Design review of the part built by this model. Coordinates are the model's own, in mm. A direction names the side the tool comes from. Give positions to 0.01 mm unless a question says otherwise; leave off trailing zeros. Use a Markdown table: item, result. Add a question column.
(1) For probe 1 along Y at (x, z) = (26.8, 6.5); probe 2 along Y at (x, z) = (45.5, 5); probe 3 along Z at (x, y) = (45, 74), list the stretches that pass through material, from the lowest coordinate up.
(2) Add section A-A, the plane z = 32. State how many separate pieces and enclosed holes the cut face has, then the cut area to 3 significant figures.
(3) Draft analysis for pull direction Z (two halves, no side actions). For faces 4 (the face through (25, 84, 25)), 5 (the face through (25, 2, 40)), 6 (the face through (33, 75, 5)), state which applies: pulls with the +Z half, pulls with the -Z half, needs draft (parallel to the pull), parting line crosses it, or undercut.
(4) Insertion check: pin 1 Ø1.8 at (x, y) = (26.8, 55.25) entering from -Z (3 decimals); pin 2 Ø1.5 at (x, y) = (30, 22.5) entering from +Z. Each pin has a flat end and moves straight along its axis. Give the tip position at first contact, or say it passes through.
(5) For faces 1 (the face through (25.524, 94.807, 4.955)), 2 (the face through (25, 68, 40)), 3 (the face through (25, 75, 25)), list the 3-axis set-ups (+Z, -Z, +X, -X, +Y, -Y) from which the entire face can be reached by the end or side of a thin tool; tool diameter is ignored.
```python
from build123d import *

# Parameters (mm, degrees)
SKETCH2_W                     = 50
SKETCH2_H                     = 100
BOSS_EXTRUDE1_DEPTH           = 40
M3_TAPPED_HOLE2_D             = 2.5
M3_TAPPED_HOLE2_DEPTH         = 10
M3_TAPPED_HOLE2_CSINK_D       = 3.05
M3_TAPPED_HOLE2_CSINK_ANGLE   = 90
M3_TAPPED_HOLE2_TIP           = 0.751075774
M2_TAPPED_HOLE1_AT_2_COUNT    = 2
M2_TAPPED_HOLE1_AT_2_PITCH    = 15.945218719
LPATTERN1_COUNT               = 3
LPATTERN1_PITCH               = 30
SKETCH6_R                     = 2
CUT_EXTRUDE4_DEPTH            = 25
M2_5_TAPPED_HOLE1_D           = 2.05
M2_5_TAPPED_HOLE1_DEPTH       = 10
M2_5_TAPPED_HOLE1_CSINK_D     = 2.55
M2_5_TAPPED_HOLE1_CSINK_ANGLE = 90
M2_5_TAPPED_HOLE1_TIP         = 0.615882135
SKETCH8_W                     = 30
SKETCH8_H                     = 3
CUT_EXTRUDE6_DEPTH            = 51
M2_TAPPED_HOLE2_D             = 1.6
M2_TAPPED_HOLE2_DEPTH         = 10
M2_TAPPED_HOLE2_CSINK_D       = 2.05
M2_TAPPED_HOLE2_CSINK_ANGLE   = 90
M2_TAPPED_HOLE2_TIP           = 0.480688495
M2_TAPPED_HOLE3_D             = 1.6
M2_TAPPED_HOLE3_DEPTH         = 10
M2_TAPPED_HOLE3_CSINK_D       = 2.05
M2_TAPPED_HOLE3_CSINK_ANGLE   = 90
M2_TAPPED_HOLE3_TIP           = 0.480688495


with BuildPart() as part:
    # Sketch2 → Boss-Extrude1 (new body)
    with BuildSketch(Plane.XY):
        with Locations((25, 50)):
            Rectangle(SKETCH2_W, SKETCH2_H)
    extrude(amount=BOSS_EXTRUDE1_DEPTH)

    # M3 Tapped Hole2
    with Locations(Plane(origin=(50, 0, 0), x_dir=(0, 0, -1), z_dir=(1, 0, 0))):
        with Locations((-5, 74), (-5, 24)):
            CounterSinkHole(M3_TAPPED_HOLE2_D / 2, M3_TAPPED_HOLE2_CSINK_D / 2, depth=M3_TAPPED_HOLE2_DEPTH, counter_sink_angle=M3_TAPPED_HOLE2_CSINK_ANGLE)
            with Locations((0, 0, -(M3_TAPPED_HOLE2_DEPTH + M3_TAPPED_HOLE2_TIP / 2))):  # 118° drill point
                Cone(0, M3_TAPPED_HOLE2_D / 2, M3_TAPPED_HOLE2_TIP, mode=Mode.SUBTRACT)

    # Sketch12 → M2 Tapped Hole1 (revolve, cut)
    with BuildSketch(Plane(origin=(26.8, 25.25, 0), x_dir=(0, 1, 0), z_dir=(1, 0, 0))):
        Polygon((0, 0), (0, 10.480688495), (0.8, 10), (0.8, 0.225), (1.025, 0), align=None)
    m2_tapped_hole1 = revolve(axis=Axis((26.8, 25.25, -6.35), (0, 0, 1)), mode=Mode.SUBTRACT)

    # M2 Tapped Hole1 at 2: M2 Tapped Hole1 ×2
    with Locations(*[Vector(-0.752576695, -0.658504608, 0) * (i * M2_TAPPED_HOLE1_AT_2_PITCH) for i in range(1, M2_TAPPED_HOLE1_AT_2_COUNT)]):
        add(m2_tapped_hole1, mode=Mode.SUBTRACT)

    # LPattern1: M2 Tapped Hole1 ×3
    with Locations(*[(0, i * LPATTERN1_PITCH, 0) for i in range(1, LPATTERN1_COUNT)]):
        add(m2_tapped_hole1, mode=Mode.SUBTRACT)

    # LPattern1 copy 1 sketch → LPattern1 copy 1 (revolve, cut)
    with BuildSketch(Plane(origin=(14.8, 44.75, 0), x_dir=(0, 1, 0), z_dir=(1, 0, 0))):
        Polygon((0, 0), (0, 10.480688495), (0.8, 10), (0.8, 0.225), (1.025, 0), align=None)
    revolve(axis=Axis((14.8, 44.75, -6.35), (0, 0, 1)), mode=Mode.SUBTRACT)

    # LPattern1 copy 2 sketch → LPattern1 copy 2 (revolve, cut)
    with BuildSketch(Plane(origin=(14.8, 74.75, 0), x_dir=(0, 1, 0), z_dir=(1, 0, 0))):
        Polygon((0, 0), (0, 10.480688495), (0.8, 10), (0.8, 0.225), (1.025, 0), align=None)
    revolve(axis=Axis((14.8, 74.75, -6.35), (0, 0, 1)), mode=Mode.SUBTRACT)

    # Sketch6 → Cut-Extrude4 (cut)
    with BuildSketch(Plane(origin=(0, 100, 0), x_dir=(1, 0, 0), z_dir=(0, 1, 0))):
        with Locations((33, -5)):
            Circle(SKETCH6_R)
    extrude(amount=-CUT_EXTRUDE4_DEPTH, mode=Mode.SUBTRACT)

    # M2.5 Tapped Hole1
    with Locations(Plane(origin=(0, 100, 0), x_dir=(1, 0, 0), z_dir=(0, 1, 0))):
        with Locations((24.5, -5)):
            CounterSinkHole(M2_5_TAPPED_HOLE1_D / 2, M2_5_TAPPED_HOLE1_CSINK_D / 2, depth=M2_5_TAPPED_HOLE1_DEPTH, counter_sink_angle=M2_5_TAPPED_HOLE1_CSINK_ANGLE)
            with Locations((0, 0, -(M2_5_TAPPED_HOLE1_DEPTH + M2_5_TAPPED_HOLE1_TIP / 2))):  # 118° drill point
                Cone(0, M2_5_TAPPED_HOLE1_D / 2, M2_5_TAPPED_HOLE1_TIP, mode=Mode.SUBTRACT)

    # Sketch8 → Cut-Extrude6 (cut, through all)
    with BuildSketch(Plane(origin=(50, 0, 0), x_dir=(0, 0, -1), z_dir=(1, 0, 0))):
        with Locations((-25, 4.5)):
            Rectangle(SKETCH8_W, SKETCH8_H)
        with Locations((-25, 10.5)):
            Rectangle(SKETCH8_W, SKETCH8_H)
        with Locations((-25, 16.5)):
            Rectangle(SKETCH8_W, SKETCH8_H)
        with Locations((-25, 22.5)):
            Rectangle(SKETCH8_W, SKETCH8_H)
        with Locations((-25, 28.5)):
            Rectangle(SKETCH8_W, SKETCH8_H)
        with Locations((-25, 34.5)):
            Rectangle(SKETCH8_W, SKETCH8_H)
        with Locations((-25, 40.5)):
            Rectangle(SKETCH8_W, SKETCH8_H)
        with Locations((-25, 46.5)):
            Rectangle(SKETCH8_W, SKETCH8_H)
        with Locations((-25, 52.5)):
            Rectangle(SKETCH8_W, SKETCH8_H)
        with Locations((-25, 58.5)):
            Rectangle(SKETCH8_W, SKETCH8_H)
        with Locations((-25, 64.5)):
            Rectangle(SKETCH8_W, SKETCH8_H)
        with Locations((-25, 70.5)):
            Rectangle(SKETCH8_W, SKETCH8_H)
        with Locations((-25, 76.5)):
            Rectangle(SKETCH8_W, SKETCH8_H)
        with Locations((-25, 82.5)):
            Rectangle(SKETCH8_W, SKETCH8_H)
        with Locations((-25, 88.5)):
            Rectangle(SKETCH8_W, SKETCH8_H)
        with Locations((-25, 94.5)):
            Rectangle(SKETCH8_W, SKETCH8_H)
    extrude(amount=-CUT_EXTRUDE6_DEPTH, mode=Mode.SUBTRACT)

    # M2 Tapped Hole2
    with Locations(Plane(origin=(0, 100, 0), x_dir=(1, 0, 0), z_dir=(0, 1, 0))):
        with Locations((15, -36), (35, -36)):
            CounterSinkHole(M2_TAPPED_HOLE2_D / 2, M2_TAPPED_HOLE2_CSINK_D / 2, depth=M2_TAPPED_HOLE2_DEPTH, counter_sink_angle=M2_TAPPED_HOLE2_CSINK_ANGLE)
            with Locations((0, 0, -(M2_TAPPED_HOLE2_DEPTH + M2_TAPPED_HOLE2_TIP / 2))):  # 118° drill point
                Cone(0, M2_TAPPED_HOLE2_D / 2, M2_TAPPED_HOLE2_TIP, mode=Mode.SUBTRACT)

    # M2 Tapped Hole3
    with Locations(Plane(origin=(0, 0, 0), x_dir=(-1, 0, 0), z_dir=(0, -1, 0))):
        with Locations((-15, -36), (-35, -36)):
            CounterSinkHole(M2_TAPPED_HOLE3_D / 2, M2_TAPPED_HOLE3_CSINK_D / 2, depth=M2_TAPPED_HOLE3_DEPTH, counter_sink_angle=M2_TAPPED_HOLE3_CSINK_ANGLE)
            with Locations((0, 0, -(M2_TAPPED_HOLE3_DEPTH + M2_TAPPED_HOLE3_TIP / 2))):  # 118° drill point
                Cone(0, M2_TAPPED_HOLE3_D / 2, M2_TAPPED_HOLE3_TIP, mode=Mode.SUBTRACT)


solid = part.part
```
Established:
| question | item | result |
|---|---|---|
| 1 | probe 1 | 0 to 24.45, 26.05 to 54.45, 56.05 to 84.45, 86.05 to 100 |
| 1 | probe 2 | 0 to 22.75, 25.25 to 72.75, 75.25 to 100 |
| 1 | probe 3 | 0 to 3.75, 6.25 to 40 |
| 2 | separate pieces | 17 |
| 2 | enclosed holes | 0 |
| 2 | area | 2,600 mm^2 |
| 3 | face 4 | needs draft |
| 3 | face 5 | pulls with the +Z half |
| 3 | face 6 | undercut |
| 4 | pin 1 | z = 0.125 |
| 4 | pin 2 | z = 10 |
| 5 | face 1 | +Y |
| 5 | face 2 | +Z, +X, -X, +Y, -Y |
| 5 | face 3 | +Z, +X, -X |
